Build history of the part. All positions in model axes, mm. A direction names the side the tool comes from. Round coordinates to 2 decimals unless told otherwise and drop trailing zeros. Loops run counter-clockwise (first coordinate to the right, second up) from the corner with the lowest first, then second, coordinate; pieces in that order, holes last. Notation, with made-up numbers: M -8,19 L 21,19 A30 ccw 21,41 Z; hole C -11,76 d4. An arc over 180 degrees is marked long. Write each question's results on one line, items separated by ' | '. Start each with the question number.
```python
from build123d import *

# Parameters (mm, degrees)
BOSS_EXTRU_1_DEPTH                  = 13
ESQUISSE2_W                         = 18.874173297
ESQUISSE2_H                         = 12.028484965
ESQUISSE2_R                         = 3
ENL_V_MAT_EXTRU_1_DEPTH             = 5
CHANFREIN1_SIZE                     = 3.25
DIAM_TRE_DU_PER_AGE_1_5_1_5_1_D     = 1.5
DIAM_TRE_DU_PER_AGE_1_5_1_5_1_DEPTH = 12.1
DIAM_TRE_DU_PER_AGE_1_5_1_5_1_TIP   = 0.450645464
DIAM_TRE_DU_PER_AGE_2_0_2_1_D       = 2
DIAM_TRE_DU_PER_AGE_2_0_2_1_DEPTH   = 10.6
DIAM_TRE_DU_PER_AGE_2_0_2_1_TIP     = 0.600860619
DIAM_TRE_DU_PER_AGE_0_4_0_4_1_D     = 0.4
DIAM_TRE_DU_PER_AGE_0_4_0_4_1_DEPTH = 1
DIAM_TRE_DU_PER_AGE_0_4_0_4_1_TIP   = 0.120172124


with BuildPart() as part:
    # Esquisse1 → Boss.-Extru.1 (new body)
    with BuildSketch(Plane.XY):
        Polygon((4.618802154, 0), (2.309401077, 4), (-2.309401077, 4), (-4.618802154, 0), (-2.309401077, -4), (2.309401077, -4), align=None)
    extrude(amount=BOSS_EXTRU_1_DEPTH)

    # Esquisse2 → Enlèv. mat.-Extru.1 (cut)
    with BuildSketch(Plane.XY.offset(13)):
        with Locations((-1.221770637, -0.072445614)):
            Rectangle(ESQUISSE2_W, ESQUISSE2_H)
        Circle(ESQUISSE2_R, mode=Mode.SUBTRACT)
    extrude(amount=-ENL_V_MAT_EXTRU_1_DEPTH, mode=Mode.SUBTRACT)

    # Chanfrein1
    chanfrein1_edges = [part.edges().sort_by_distance(p)[0] for p in [
        (0, -4, 0),
        (-3.464101615, -2, 0),
        (-3.464101615, 2, 0),
        (0, 4, 0),
        (3.464101615, 2, 0),
        (3.464101615, -2, 0),
    ]]
    chamfer(chanfrein1_edges, length=CHANFREIN1_SIZE)

    # Diamètre du perçage Ø1.5 (1.5)1
    with Locations(Plane.XY.offset(13)):
        with Locations((0, 0)):
            Hole(DIAM_TRE_DU_PER_AGE_1_5_1_5_1_D / 2, depth=DIAM_TRE_DU_PER_AGE_1_5_1_5_1_DEPTH)
            with Locations((0, 0, -(DIAM_TRE_DU_PER_AGE_1_5_1_5_1_DEPTH + DIAM_TRE_DU_PER_AGE_1_5_1_5_1_TIP / 2))):  # 118° drill point
                Cone(0, DIAM_TRE_DU_PER_AGE_1_5_1_5_1_D / 2, DIAM_TRE_DU_PER_AGE_1_5_1_5_1_TIP, mode=Mode.SUBTRACT)

    # Diamètre du perçage Ø2.0 (2)1
    with Locations(Plane.XY.offset(13)):
        with Locations((0, 0)):
            Hole(DIAM_TRE_DU_PER_AGE_2_0_2_1_D / 2, depth=DIAM_TRE_DU_PER_AGE_2_0_2_1_DEPTH)
            with Locations((0, 0, -(DIAM_TRE_DU_PER_AGE_2_0_2_1_DEPTH + DIAM_TRE_DU_PER_AGE_2_0_2_1_TIP / 2))):  # 118° drill point
                Cone(0, DIAM_TRE_DU_PER_AGE_2_0_2_1_D / 2, DIAM_TRE_DU_PER_AGE_2_0_2_1_TIP, mode=Mode.SUBTRACT)

    # Diamètre du perçage Ø0.4 (0.4)1
    with Locations(Plane(origin=(0, 0, 0), x_dir=(-1, 0, 0), z_dir=(0, 0, -1))):
        with Locations((0, 0)):
            Hole(DIAM_TRE_DU_PER_AGE_0_4_0_4_1_D / 2, depth=DIAM_TRE_DU_PER_AGE_0_4_0_4_1_DEPTH)
            with Locations((0, 0, -(DIAM_TRE_DU_PER_AGE_0_4_0_4_1_DEPTH + DIAM_TRE_DU_PER_AGE_0_4_0_4_1_TIP / 2))):  # 118° drill point
                Cone(0, DIAM_TRE_DU_PER_AGE_0_4_0_4_1_D / 2, DIAM_TRE_DU_PER_AGE_0_4_0_4_1_TIP, mode=Mode.SUBTRACT)


solid = part.part
```
Item 1: Mould opens along X. For faces 1 (the flat face through (3.48, 1.97, 5.59)), 2 (the flat face through (-0.03, -2.76, 2.01)), 3 (the flat face through (-3.448, 2.028, 5.592)), 4 (the cylindrical face through (0.75, 0.03, 1.57)) say: released by +X, released by -X, zero draft, split by the parting line, or undercut.
Item 2: Tool access for faces 5 (the cylindrical face through (-3, 0, 11)), 6 (the flat face through (2.366, 1.329, 1.963)): list every direction of +Z, -Z, +X, -X, +Y, -Y with a clear straight run to the whole face (end or side of a thin tool).
Item 3: Saw through at C-C, the plane y = -2. Give the cut face in (x, z).
Item 4: Saw through at B-B, the plane z = 7. Give the cut face in (x, y), then the cut area to 3 significant figures.
Item 5: Saw through at D-D, the plane x = 1.75. Give the cut face in (y, z).
Item 6: Saw through at A-A, the plane x = 0. Give the cut face in (y, z).
Item 7: Drop flat-ended pins along their axis: pin 1 (2 mm diameter, centred on x = -3, y = -1, fed in from +Z); pin 2 (2 mm diameter, centred on x = 3.5, z = 11, fed in from +Y); pin 3 (1.5 mm diameter, centred on x = 1.5, z = 10.5, fed in from +Y). Give the stop position or say it passes through.
Item 8: Drill centre lines: line 1 along Z through (x, y) = (-0.5, 3); line 2 along Y through (x, z) = (0.25, 6.5). Where is each one in solid material? Low to high. Write a range as [from, to].
Working result:
1) face 1: released by +X | face 2: zero draft | face 3: released by -X | face 4: undercut
2) face 5: +Z | face 6: -Z, +X, +Y
3) outline: M -3.46,3.25 L -1.15,1.25 L 1.15,1.25 L 3.46,3.25 L 3.46,8 L 2.24,8 L 2.24,13 L -2.24,13 L -2.24,8 L -3.46,8 Z
4) outline: M -4.62,0 L -2.31,-4 L 2.31,-4 L 4.62,0 L 2.31,4 L -2.31,4 Z; hole C 0,0 d2 | area: 52.3 mm²
5) outline: M -4,3.25 L -3.03,2.28 L 0,0.77 L 3.03,2.28 L 4,3.25 L 4,8 L 2.44,8 L 2.44,13 L -2.44,13 L -2.44,8 L -4,8 Z
6) outline: M -4,3.25 L -0.75,0 L -0.2,0 L -0.2,0.57 L -0.75,0.9 L -0.75,2.25 L -1,2.4 L -1,13 L -3,13 L -3,8 L -4,8 Z; M 0.2,0 L 0.75,0 L 4,3.25 L 4,8 L 3,8 L 3,13 L 1,13 L 1,2.4 L 0.75,2.25 L 0.75,0.9 L 0.2,0.57 Z
7) pin 1: stops at z = 13 | pin 2: stops at y = 1.66 | pin 3: stops at y = 2.9
8) line 1: z = [2.25, 8] | line 2: y = [-4, -0.97], [0.97, 4]
